```python
from build123d import *

# Parameters (mm, degrees)
F0_W     = 15.25
F0_H     = 6
F0_W_2   = 14.25
F0_H_2   = 5
F1_DEPTH = 32.5
F2_W     = 15.25
F2_H     = 6
F3_DEPTH = 0.5
F4_W     = 4
F4_H     = 3
F5_DEPTH = 33.001


with BuildPart() as f1:
    # F0 (on Front) → F1 (new body)
    with BuildSketch(Plane.XZ):
        Rectangle(F0_W, F0_H)
        Rectangle(F0_W_2, F0_H_2, mode=Mode.SUBTRACT)
    extrude(amount=F1_DEPTH)

    # F2 (on face) → F3 (join)
    with BuildSketch(Plane(origin=(0, 0, 0), x_dir=(-1, 0, 0), z_dir=(0, 1, 0))):
        Rectangle(F2_W, F2_H)
    extrude(amount=F3_DEPTH)

    # F4 (on face) → F5 (cut, through all)
    with BuildSketch(Plane(origin=(0, 0.5, 0), x_dir=(-1, 0, 0), z_dir=(0, 1, 0))):
        Rectangle(F4_W, F4_H)
    extrude(amount=-F5_DEPTH, mode=Mode.SUBTRACT)


solid = f1.part
```
Read the model definition and answer for the solid it produces. Units are mm, in the model's axes. A direction names the side the tool comes from. Coordinates: 2 decimals unless noted, no trailing zeros. Write each loop counter-clockwise with the first axis right and the second up, starting at its lowest first coordinate (ties: lowest second). Pieces come first, ordered by that corner, then holes. Notation, with made-up numbers: (-0.75, -40) -> (48.25, -40) arc R20 ccw to (48.25, -26) -> close; hole circle Ø6 at (-22.5, 29). An arc over 180 degrees is marked (long way). Answer as a JSON object with one key per item and string values.
Q1. The part is cut by section A-A on x = 0.5. Give the vertices of the cut face in (y, z), then the cut area to 3 significant figures.
The answers:
{"outline": "(-32.5, -3) -> (0.5, -3) -> (0.5, -1.5) -> (0, -1.5) -> (0, -2.5) -> (-32.5, -2.5) -> close; (-32.5, 2.5) -> (0, 2.5) -> (0, 1.5) -> (0.5, 1.5) -> (0.5, 3) -> (-32.5, 3) -> close", "area": "34.0 mm2"}
Q2. The part is cut by section C-C on y = -25.5. Give the vertices of the cut face in (x, z) (3 decimals), then the cut area to 4 significant figures.
The answers:
{"outline": "(-7.625, -3) -> (7.625, -3) -> (7.625, 3) -> (-7.625, 3) -> close; hole (-7.125, -2.5) -> (7.125, -2.5) -> (7.125, 2.5) -> (-7.125, 2.5) -> close", "area": "20.25 mm2"}
Q3. A tool of negligible diameter and unlimited length cuts with its end or side. For faces 1 (the flat face through (0, -16, -2.5)), 2 (the flat face through (0, -16, 3)), from which of +Z, -Z, +X, -X, +Y, -Y can it reach the whole face along a straight path? Write none if from no direction.
The answers:
{"face 1": "-Y", "face 2": "+Z, +X, -X, +Y, -Y"}
Q4. Flat-ended cylindrical pins translate along their axes: pin 1 Ø2.5 at (x, z) = (-0.5, 0.5) entering from -Y; pin 2 Ø1.5 at (x, z) = (-1.5, -0.5) entering from +Y. Find the tip coordinate at first contact, or state that the pin passes through.
The answers:
{"pin 1": "stops at y = 0", "pin 2": "stops at y = 0.5"}
Q5. The part is cut by section B-B on z = -1.2. Give the vertices of the cut face in (x, y) (3 decimals).
The answers:
{"outline": "(-7.625, -32.5) -> (-7.125, -32.5) -> (-7.125, 0) -> (-2, 0) -> (-2, 0.5) -> (-7.625, 0.5) -> close; (2, 0) -> (7.125, 0) -> (7.125, -32.5) -> (7.625, -32.5) -> (7.625, 0.5) -> (2, 0.5) -> close"}
Q6. Determine the mould class of faces 3 (the flat face through (-7.125, -16, 0)), 4 (the flat face through (0, 0.5, 2)), 5 (the flat face through (-7.625, -16, 0)) for opening direction X: pulls with the +X half, pulls with the -X half, needs draft (parallel to the pull), parting line crosses it, or undercut.
The answers:
{"face 3": "undercut", "face 4": "needs draft", "face 5": "pulls with the -X half"}
Q7. The part is cut by section D-D on x = 3. Give the vertices of the cut face in (y, z).
The answers:
{"outline": "(-32.5, -3) -> (0.5, -3) -> (0.5, 3) -> (-32.5, 3) -> (-32.5, 2.5) -> (0, 2.5) -> (0, -2.5) -> (-32.5, -2.5) -> close"}
Q8. Consider line 1 (X direction, y = -18.5, z = -1.05) (3 decimals); line 2 (Z direction, x = 3.25, y = -28.5); line 3 (Y direction, x = 5.25, z = -2.45). Determine where each line is inside the solid, lowest interval first. Write a range as [from, to].
The answers:
{"line 1": "x = [-7.625, -7.125], [7.125, 7.625]", "line 2": "z = [-3, -2.5], [2.5, 3]", "line 3": "y = [0, 0.5]"}
